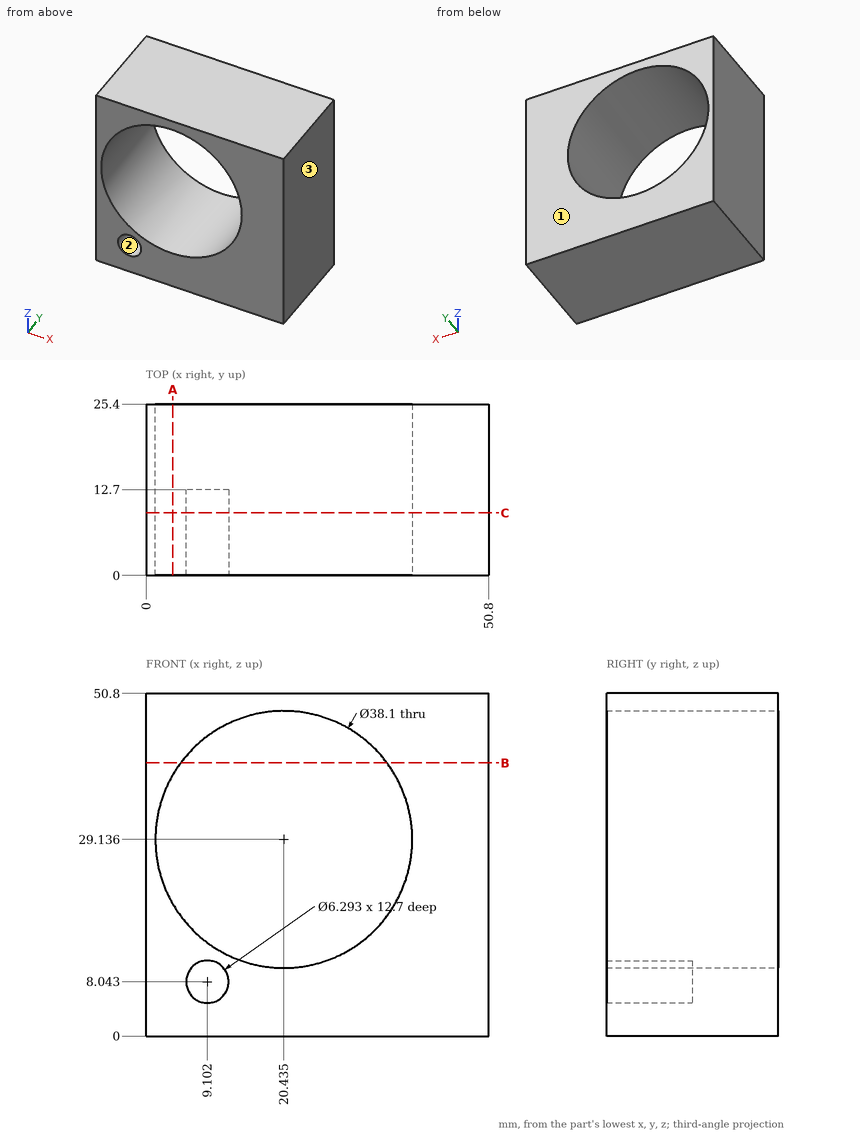
Design review of the part shown in the three views and the two pictorial views. Dimensions are in mm from the part's minimum x, y and z. Coordinates: 2 decimals unless noted, no trailing zeros. Write each loop counter-clockwise with the first axis right and the second up, starting at its lowest first coordinate (ties: lowest second). Pieces come first, ordered by that corner, then holes.
1) The part is to be moulded in two halves that separate along X. For the marked faces 1, 2 and 3, say which applies: pulls with the +X half, pulls with the -X half, needs draft (parallel to the pull), parting line crosses it, or undercut.
2) We need section B-B on z = 40.5. State the section outline as (x, y) points (1 decimal).
3) We need section A-A on x = 4. State the section outline as (y, z) points (1 decimal), then the cut area to 3 significant figures.
4) To check wall thickness, follow probe 1 along Z at (x, y) = (24, 18.25); probe 2 along Z at (x, y) = (26, 22.25) (1 decimal); probe 3 along X at (y, z) = (11, 34) (1 decimal). State the ranges of each line that lie inside material, in increasing order.
5) We need section C-C on y = 9.25. Count the separate pieces of the cut face and the enclosed holes in it, then the cut area to 3 significant figures.
6) Clearance check with flat-ended pins moving along their axes: pin 1 Ø12 at (y, z) = (7.5, 37) entering from -X; pin 2 Ø5 at (x, z) = (9.1, 8.04) entering from -Y. State where each tip first meets the part, or that it passes through.
Answer list:
1. face 1: needs draft
1. face 2: undercut
1. face 3: pulls with the +X half
2. outline: (0, 0) - (5.1, 0) - (5.1, 25.4) - (0, 25.4) - close; (35.7, 0) - (50.8, 0) - (50.8, 25.4) - (35.7, 25.4) - close
3. outline: (0, 0) - (25.4, 0) - (25.4, 19.5) - (0, 19.5) - close; (0, 38.8) - (25.4, 38.8) - (25.4, 50.8) - (0, 50.8) - close
3. area: 801 mm2
4. probe 1: z = 0 to 10.42, 47.85 to 50.8
4. probe 2: z = 0 to 10.9, 47.4 to 50.8
4. probe 3: x = 0 to 2, 38.9 to 50.8
5. separate pieces: 1
5. enclosed holes: 2
5. area: 1,410 mm2
6. pin 1: stops at x = 0
6. pin 2: stops at y = 12.7
